Build history of the part. All positions in model axes, mm. Give positions to 0.01 mm unless a question says otherwise; leave off trailing zeros. Loops run counter-clockwise (first coordinate to the right, second up) from the corner with the lowest first, then second, coordinate; pieces in that order, holes last. Notation, with made-up numbers: (17, 0) -> (42, 0) arc R36 ccw to (42, 35) -> close; hole circle Ø7 at (79.5, 82.25). An arc over 180 degrees is marked (long way). Answer in a Markdown table with one row per item. Add a question column.
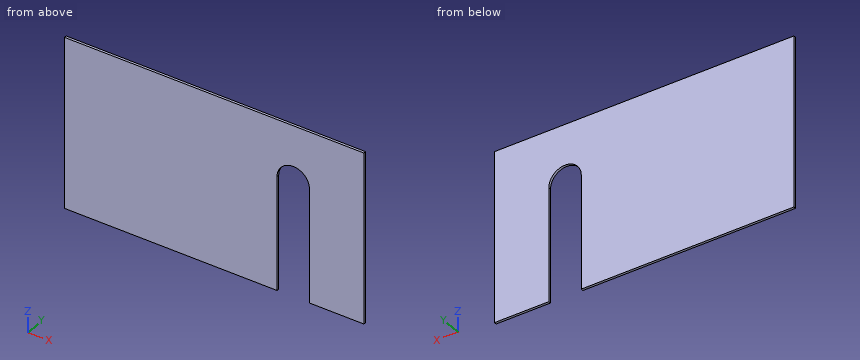
from build123d import *

# Parameters (mm, degrees)
F1_DEPTH = 6


with BuildPart() as f1:
    # F0 (on Front) → F1 (new body)
    with BuildSketch(Plane.XZ):
        with BuildLine():
            Line((0, 420), (0, 0))
            Line((0, 0), (524, 0))
            Line((524, 0), (524, 280))
            ThreePointArc((524, 280), (564, 320), (604, 280))
            Line((604, 280), (604, 0))
            Line((604, 0), (738, 0))
            Line((738, 0), (738, 420))
            Line((738, 420), (0, 420))
        make_face()
    extrude(amount=F1_DEPTH)


solid = f1.part
(1) Saw through at A-A, the plane z = 119. List the corners of the cut face in (x, y), then the cut area to 3 significant figures.
(2) Saw through at B-B, the plane y = -3.75. List the corners of the cut face in (x, z), then the cut area to 3 significant figures.
(3) Saw through at C-C, the plane x = 564. List the corners of the cut face in (y, z).
(4) Wall check: line 1 along X through (y, z) = (-4.2, 248); line 2 along X through (y, z) = (-1.85, 317); line 3 along Z through (x, y) = (592, -4.65). Give the ranges that are in metal, low to high. Write a range as from..to.
Worked answers:
| question | item | result |
|---|---|---|
| 1 | outline | (0, -6) -> (524, -6) -> (524, 0) -> (0, 0) -> close; (604, -6) -> (738, -6) -> (738, 0) -> (604, 0) -> close |
| 1 | area | 3,950 mm^2 |
| 2 | outline | (0, 0) -> (524, 0) -> (524, 280) arc R40 cw to (604, 280) -> (604, 0) -> (738, 0) -> (738, 420) -> (0, 420) -> close |
| 2 | area | 285,000 mm^2 |
| 3 | outline | (-6, 320) -> (0, 320) -> (0, 420) -> (-6, 420) -> close |
| 4 | line 1 | 0..524, 604..738 |
| 4 | line 2 | 0..548.8, 579.2..738 |
| 4 | line 3 | 308.57..420 |
